```python
from build123d import *

# Parameters (mm, degrees)
ESTRUSIONE_ESTRUSIONE1_DEPTH = 300
SCHIZZO2_W                   = 3.5
SCHIZZO2_H                   = 4.6
TAGLIO_ESTRUSIONE1_DEPTH     = 303.096048468


with BuildPart() as part:
    # Schizzo1 → Estrusione-Estrusione1 (new body)
    with BuildSketch(Plane.XY):
        with BuildLine():
            Line((-30.15, 14), (-32.65, 14))
            Line((-32.65, 14), (-32.65, 8.9))
            Line((-32.65, 8.9), (-30.45, 8.9))
            Line((-30.45, 8.9), (-30.45, 7.8))
            Line((-30.45, 7.8), (-20.55, 7.8))
            Line((-20.55, 7.8), (-20.55, 0))
            Line((-20.55, 0), (-30.45, 0))
            Line((-30.45, 0), (-30.45, -2.2))
            Line((-30.45, -2.2), (-32.65, -2.2))
            Line((-32.65, -2.2), (-32.65, -5.3))
            Line((-32.65, -5.3), (-31.15, -5.3))
            Line((-31.15, -5.3), (-31.15, -3.3))
            Line((-31.15, -3.3), (-28.75, -3.3))
            Line((-28.75, -3.3), (-28.75, -5.3))
            Line((-28.75, -5.3), (-25.45, -5.3))
            Line((-25.45, -5.3), (-25.45, -3.8))
            Line((-25.45, -3.8), (-27.25, -3.8))
            Line((-27.25, -3.8), (-27.25, -1.8))
            Line((-27.25, -1.8), (-22.05, -1.8))
            Line((-22.05, -1.8), (-22.05, -5.3))
            Line((-22.05, -5.3), (-18.85, -5.3))
            Line((-18.85, -5.3), (-18.85, 7.8))
            Line((-18.85, 7.8), (-15.821542758, 7.8))
            ThreePointArc((-15.821542758, 7.8), (-16.273540604, 4.846345824), (-14.423395659, 2.5))
            Line((-14.423395659, 2.5), (-14.074102014, 2.5))
            Line((-14.074102014, 2.5), (-14.074102014, 4.405182935))
            ThreePointArc((-14.074102014, 4.405182935), (-12.647585955, 7.8), (-11.221069895, 4.405182935))
            Line((-11.221069895, 4.405182935), (-11.221069895, 2.5))
            Line((-11.221069895, 2.5), (-10.87177625, 2.5))
            ThreePointArc((-10.87177625, 2.5), (-9.021631305, 4.846345824), (-9.473629151, 7.8))
            Line((-9.473629151, 7.8), (0, 7.8))
            Line((0, 7.8), (0, 9.4))
            Line((0, 9.4), (-29.15, 9.4))
            Line((-29.15, 9.4), (-29.15, 10.5))
            Line((-29.15, 10.5), (-30.15, 10.5))
            Line((-30.15, 10.5), (-30.15, 14))
        make_face()
        with BuildLine():
            Line((29.15, 9.4), (0, 9.4))
            Line((0, 9.4), (0, 7.8))
            Line((0, 7.8), (9.473629151, 7.8))
            ThreePointArc((9.473629151, 7.8), (9.021631305, 4.846345824), (10.87177625, 2.5))
            Line((10.87177625, 2.5), (11.221069895, 2.5))
            Line((11.221069895, 2.5), (11.221069895, 4.405182935))
            ThreePointArc((11.221069895, 4.405182935), (12.647585955, 7.8), (14.074102014, 4.405182935))
            Line((14.074102014, 4.405182935), (14.074102014, 2.5))
            Line((14.074102014, 2.5), (14.423395659, 2.5))
            ThreePointArc((14.423395659, 2.5), (16.273540604, 4.846345824), (15.821542758, 7.8))
            Line((15.821542758, 7.8), (18.85, 7.8))
            Line((18.85, 7.8), (18.85, -5.3))
            Line((18.85, -5.3), (22.05, -5.3))
            Line((22.05, -5.3), (22.05, -1.8))
            Line((22.05, -1.8), (27.25, -1.8))
            Line((27.25, -1.8), (27.25, -3.8))
            Line((27.25, -3.8), (25.45, -3.8))
            Line((25.45, -3.8), (25.45, -5.3))
            Line((25.45, -5.3), (28.75, -5.3))
            Line((28.75, -5.3), (28.75, -3.3))
            Line((28.75, -3.3), (31.15, -3.3))
            Line((31.15, -3.3), (31.15, -5.3))
            Line((31.15, -5.3), (32.65, -5.3))
            Line((32.65, -5.3), (32.65, -2.2))
            Line((32.65, -2.2), (30.45, -2.2))
            Line((30.45, -2.2), (30.45, 0))
            Line((30.45, 0), (20.55, 0))
            Line((20.55, 0), (20.55, 7.8))
            Line((20.55, 7.8), (30.45, 7.8))
            Line((30.45, 7.8), (30.45, 8.9))
            Line((30.45, 8.9), (32.65, 8.9))
            Line((32.65, 8.9), (32.65, 14))
            Line((32.65, 14), (30.15, 14))
            Line((30.15, 14), (30.15, 10.5))
            Line((30.15, 10.5), (29.15, 10.5))
            Line((29.15, 10.5), (29.15, 9.4))
        make_face()
    extrude(amount=ESTRUSIONE_ESTRUSIONE1_DEPTH)

    # Schizzo2 → Taglio-Estrusione1 (cut, through all)
    with BuildSketch(Plane.XY.offset(300)):
        with Locations((30.9, 11.7)):
            Rectangle(SCHIZZO2_W, SCHIZZO2_H)
    taglio_estrusione1 = extrude(amount=-TAGLIO_ESTRUSIONE1_DEPTH, mode=Mode.SUBTRACT)

    # Specchia1: Taglio-Estrusione1 across plane
    add(taglio_estrusione1.mirror(Plane(origin=(0, 0, 0), x_dir=(0, 0, 1), z_dir=(1, 0, 0))), mode=Mode.SUBTRACT)


solid = part.part
```
Work out the finished part from the listing and answer in its coordinate system (mm). A direction names the side the tool comes from. Round coordinates to 2 decimals unless told otherwise and drop trailing zeros. Loops run counter-clockwise (first coordinate to the right, second up) from the corner with the lowest first, then second, coordinate; pieces in that order, holes last.
(1) The mould has two halves that part along Y. Classify faces 4 (the flat face through (25, -1.8, 148)), 5 (the flat face through (-18.85, 1, 148)), 6 (the flat face through (0, 9.4, 152)): pulls with the +Y half, pulls with the -Y half, needs draft (parallel to the pull), parting line crosses it, or undercut.
Computed values:
face 4: undercut
face 5: needs draft
face 6: pulls with the +Y half
(2) For faces 1 (the flat face through (-25, -1.8, 148)), 2 (the flat face through (-20.55, 4, 148)), 3 (the flat face through (18.85, 1, 148)), determine the directions among +Z, -Z, +X, -X, +Y, -Y from which every point of the face is accessible in a straight line to the end or side of a thin tool.
Computed values:
face 1: +Z, -Z
face 2: +Z, -Z, -X
face 3: +Z, -Z, -Y
(3) The part is cut by section A-A, the plane x = -2. Give the vertices of the cut face in (y, z), and give its area (3 significant figures).
Computed values:
outline: (7.8, 0) - (9.4, 0) - (9.4, 300) - (7.8, 300) - close
area: 480 mm2
(4) Each of these flat-tipped pins is pushed along its axis until it touches: P1, Ø2, axis at y = 3.5, z = 91, coming from the -X side; P2, Ø2, axis at y = 3.5, z = 129, coming from the +X side; P3, Ø1.5, axis at x = 25.5, y = 6, coming from the +Z side; P4, Ø1.8, axis at y = -0.5, z = 90, coming from the -X side. Where does it stop, or does it pass through?
Computed values:
P1: stops at x = -20.55
P2: stops at x = 20.55
P3: passes through
P4: stops at x = -30.45
(5) Find the intervals of material crossed by L1, parallel to X at y = 6, z = 74; L2, parallel to X at y = -4.25, z = 226; L3, parallel to Y at x = 26.5, z = 184.5, in increasing order.
Computed values:
L1: x = -20.55 to -18.85, -16.39 to -14.63, -10.66 to -8.9, 8.9 to 10.66, 14.63 to 16.39, 18.85 to 20.55
L2: x = -32.65 to -31.15, -28.75 to -25.45, -22.05 to -18.85, 18.85 to 22.05, 25.45 to 28.75, 31.15 to 32.65
L3: y = -5.3 to -3.8, -1.8 to 0, 7.8 to 9.4
